Geometry: final body of the model. Coordinates: model frame, mm. A direction names the side the tool comes from. Give positions to 0.01 mm unless a question says otherwise; leave off trailing zeros. Write each loop counter-clockwise with the first axis right and the second up, starting at its lowest first coordinate (ties: lowest second). Pieces come first, ordered by that corner, then holes.
from build123d import *

# Parameters (mm, degrees)
SKETCH2_R           = 50
SKETCH2_R_2         = 2.5
SKETCH2_R_3         = 2
BOSS_EXTRUDE1_DEPTH = 3


with BuildPart() as part:
    # Sketch2 → Boss-Extrude1 (new body)
    with BuildSketch(Plane(origin=(0, 0, 0), x_dir=(1, 0, 0), z_dir=(0, 1, 0))):
        with Locations(Location((0, 0, 0), (0, 0, 270))):
            Circle(SKETCH2_R)
        with Locations(Location((-24.748737342, 24.748737342, 0), (0, 0, 270))):
            Circle(SKETCH2_R_2, mode=Mode.SUBTRACT)
        with Locations(Location((24.748737342, 24.748737342, 0), (0, 0, 270))):
            Circle(SKETCH2_R_2, mode=Mode.SUBTRACT)
        with Locations(Location((24.748737342, -24.748737342, 0), (0, 0, 270))):
            Circle(SKETCH2_R_2, mode=Mode.SUBTRACT)
        with Locations(Location((-24.748737342, -24.748737342, 0), (0, 0, 270))):
            Circle(SKETCH2_R_2, mode=Mode.SUBTRACT)
        with Locations(Location((15.772078615, 5, 0), (0, 0, 270))):
            Circle(SKETCH2_R_3, mode=Mode.SUBTRACT)
        with Locations(Location((15.772078615, -5, 0), (0, 0, 90))):
            Circle(SKETCH2_R_3, mode=Mode.SUBTRACT)
        with Locations(Location((-35.316235845, -5, 0), (0, 0, 270))):
            Circle(SKETCH2_R_3, mode=Mode.SUBTRACT)
        with Locations(Location((-35.316235845, 5, 0), (0, 0, 90))):
            Circle(SKETCH2_R_3, mode=Mode.SUBTRACT)
        Polygon((-9.772078615, -10), (9.772078615, -10), (9.772078615, 10), (-9.772078615, 10), (-30.227921385, 10), (-30.227921385, -10), align=None, mode=Mode.SUBTRACT)
    extrude(amount=BOSS_EXTRUDE1_DEPTH)


solid = part.part
Q1. Pull-direction query (Z, two-part tool) for faces 1 (the cylindrical face through (14.42, 1.479, 6.474)), 2 (the cylindrical face through (15.02, 1.48, 47.69)), 3 (the flat face through (0.7, 0, 10.4)); classes: released by +Z, released by -Z, zero draft, split by the parting line, or undercut.
Filled sheet:
face 1: undercut
face 2: split by the parting line
face 3: zero draft
Q2. Ray query, line 1 along X through (y, z) = (1.2, -23); line 2 along X through (y, z) = (2.05, 5); line 3 along X through (y, z) = (1.9, 26). Return the intervals inside material, ascending.
Filled sheet:
line 1: x = -44.4 to -26.54, -22.96 to 22.96, 26.54 to 44.4
line 2: x = -49.75 to -37.32, -33.32 to -30.23, 9.77 to 13.77, 17.77 to 49.75
line 3: x = -42.71 to -26.91, -22.58 to 22.58, 26.91 to 42.71
Q3. Section A-A on z = 0. Output: boundary loops of the cut face in (x, y), plus the area to 3 significant figures.
Filled sheet:
outline: (-50, 0) - (-30.23, 0) - (-30.23, 3) - (-50, 3) - close; (9.77, 0) - (50, 0) - (50, 3) - (9.77, 3) - close
area: 180 mm2
Q4. Section D-D on z = 39. Output: boundary loops of the cut face in (x, y).
Filled sheet:
outline: (-31.29, 0) - (31.29, 0) - (31.29, 3) - (-31.29, 3) - close
Q5. Access query for faces 4 (the flat face through (9.772, 1, 0)), 5 (the flat face through (0.7, 3, 10.4)). Directions: +Z, -Z, +X, -X, +Y, -Y. A direction counts if a zero-diameter tool reaches every point of the face in a straight line with its end or side. Return the directions, or none.
Filled sheet:
face 4: +Y, -Y
face 5: +Z, -Z, +X, -X, +Y
Q6. Section B-B on x = 0. Output: boundary loops of the cut face in (y, z).
Filled sheet:
outline: (0, -50) - (3, -50) - (3, -10) - (0, -10) - close; (0, 10) - (3, 10) - (3, 50) - (0, 50) - close
Q7. Section C-C on y = 1.8. Count the separate pieces of the cut face and the enclosed holes in it, plus the area to 3 significant figures.
Filled sheet:
separate pieces: 1
enclosed holes: 9
area: 6,930 mm2
Q8. Pin query (flat end, axial travel): P1, Ø1, axis at x = -26, y = 0.5, coming from the -Z side; P2, Ø0.9, axis at x = -15, y = 1, coming from the -Z side; P3, Ø1.5, axis at y = 2.5, z = -16.5, coming from the +X side. Return the tip coordinate at first contact, or that it passes through.
Filled sheet:
P1: stops at z = -43.01
P2: stops at z = -47.84
P3: stops at x = 47.45
